Geometry: final body of the model. Coordinates: model frame, mm. Give positions to 0.01 mm unless a question says otherwise; leave off trailing zeros. Order: outer loops, then holes, each group sorted by start corner. A loop starts at its lowest first (then second) coordinate and runs counter-clockwise, first axis right, second up. Notation, with made-up numbers: (-38.5, -27.75) -> (-1.5, -27.75) arc R19 ccw to (-1.5, 1.25) -> close; hole circle Ø4 at (79.5, 29). An arc over 180 degrees is marked (long way). Write item = value, one per line.
```python
from build123d import *

# Parameters (mm, degrees)
SKETCH1_W           = 368.3
SKETCH1_H           = 127
SKETCH1_R           = 2.032
BOSS_EXTRUDE1_DEPTH = 3.175
FILLET1_R           = 5.08
FILLET3_R           = 6.35
FILLET4_R           = 2.54
FILLET5_R           = 6.35
CUT_EXTRUDE1_REACH  = 196.817
SKETCH2_R           = 2.032


with BuildPart() as part:
    # Sketch1 → Boss-Extrude1 (new body)
    with BuildSketch(Plane(origin=(0, 0, 0), x_dir=(1, 0, 0), z_dir=(0, 1, 0))):
        Rectangle(SKETCH1_W, SKETCH1_H)
        with Locations(Location((-171.45, -57.15, 0), (0, 0, 270))):
            Circle(SKETCH1_R, mode=Mode.SUBTRACT)
        with Locations(Location((-146.05, -57.15, 0), (0, 0, 270))):
            Circle(SKETCH1_R, mode=Mode.SUBTRACT)
        with Locations(Location((-95.25, -45.0215, 0), (0, 0, 270))):
            Circle(SKETCH1_R, mode=Mode.SUBTRACT)
        with Locations(Location((-82.55, -45.0215, 0), (0, 0, 270))):
            Circle(SKETCH1_R, mode=Mode.SUBTRACT)
        with Locations(Location((-60.9677978, -44.45, 0), (0, 0, 270))):
            Circle(SKETCH1_R, mode=Mode.SUBTRACT)
        with Locations(Location((-48.2677978, -44.45, 0), (0, 0, 270))):
            Circle(SKETCH1_R, mode=Mode.SUBTRACT)
        with Locations(Location((-154.94, -18.415, 0), (0, 0, 270))):
            Circle(SKETCH1_R, mode=Mode.SUBTRACT)
        with Locations(Location((-142.24, -18.415, 0), (0, 0, 270))):
            Circle(SKETCH1_R, mode=Mode.SUBTRACT)
        with Locations(Location((2.1088604, -44.45, 0), (0, 0, 270))):
            Circle(SKETCH1_R, mode=Mode.SUBTRACT)
        with Locations(Location((14.8088604, -44.45, 0), (0, 0, 270))):
            Circle(SKETCH1_R, mode=Mode.SUBTRACT)
        with Locations(Location((158.3188604, -44.45, 0), (0, 0, 270))):
            Circle(SKETCH1_R, mode=Mode.SUBTRACT)
        with Locations(Location((171.0188604, -44.45, 0), (0, 0, 270))):
            Circle(SKETCH1_R, mode=Mode.SUBTRACT)
        Polygon((-134.618428208, -13.335), (-165.098428208, -13.335), (-165.098428208, 40.005), (-134.618428208, 40.005), (-134.618428208, 26.67), (-126.998428208, 26.67), (-126.998428208, 0), (-134.618428208, 0), align=None, mode=Mode.SUBTRACT)
        with Locations(Location((-60.9677978, 0, 0), (0, 0, 270))):
            Circle(SKETCH1_R, mode=Mode.SUBTRACT)
        with Locations(Location((-48.2677978, 0, 0), (0, 0, 270))):
            Circle(SKETCH1_R, mode=Mode.SUBTRACT)
        with Locations(Location((-171.45, 57.15, 0), (0, 0, 270))):
            Circle(SKETCH1_R, mode=Mode.SUBTRACT)
        with Locations(Location((-146.05, 57.15, 0), (0, 0, 270))):
            Circle(SKETCH1_R, mode=Mode.SUBTRACT)
        with Locations(Location((-60.9677978, 44.45, 0), (0, 0, 270))):
            Circle(SKETCH1_R, mode=Mode.SUBTRACT)
        with Locations(Location((-48.2677978, 44.45, 0), (0, 0, 270))):
            Circle(SKETCH1_R, mode=Mode.SUBTRACT)
        with Locations(Location((2.1088604, 0, 0), (0, 0, 270))):
            Circle(SKETCH1_R, mode=Mode.SUBTRACT)
        with Locations(Location((14.8088604, 0, 0), (0, 0, 270))):
            Circle(SKETCH1_R, mode=Mode.SUBTRACT)
        with Locations(Location((158.3188604, 0, 0), (0, 0, 270))):
            Circle(SKETCH1_R, mode=Mode.SUBTRACT)
        with Locations(Location((171.0188604, 0, 0), (0, 0, 270))):
            Circle(SKETCH1_R, mode=Mode.SUBTRACT)
        with Locations(Location((2.1088604, 44.45, 0), (0, 0, 270))):
            Circle(SKETCH1_R, mode=Mode.SUBTRACT)
        with Locations(Location((14.8088604, 44.45, 0), (0, 0, 270))):
            Circle(SKETCH1_R, mode=Mode.SUBTRACT)
        with Locations(Location((158.3188604, 44.45, 0), (0, 0, 270))):
            Circle(SKETCH1_R, mode=Mode.SUBTRACT)
        with Locations(Location((171.0188604, 44.45, 0), (0, 0, 270))):
            Circle(SKETCH1_R, mode=Mode.SUBTRACT)
    extrude(amount=BOSS_EXTRUDE1_DEPTH)

    # Fillet1
    fillet1_edges = [part.edges().sort_by_distance(p)[0] for p in [
        (-134.618428208, 1.5875, -40.005),
        (-165.098428208, 1.5875, -40.005),
        (-165.098428208, 1.5875, 13.335),
        (-134.618428208, 1.5875, 13.335),
    ]]
    fillet(fillet1_edges, radius=FILLET1_R)

    # Fillet3
    fillet3_edges = [part.edges().sort_by_distance(p)[0] for p in [
        (184.15, 1.5875, -63.5),
        (184.15, 1.5875, 63.5),
        (-184.15, 1.5875, 63.5),
        (-184.15, 1.5875, -63.5),
    ]]
    fillet(fillet3_edges, radius=FILLET3_R)

    # Fillet4
    fillet4_edges = [part.edges().sort_by_distance(p)[0] for p in [
        (-126.998428208, 1.5875, -26.67),
        (-126.998428208, 1.5875, 0),
    ]]
    fillet(fillet4_edges, radius=FILLET4_R)

    # Fillet5
    fillet5_edges = [part.edges().sort_by_distance(p)[0] for p in [
        (-134.618428208, 1.5875, 0),
        (-134.618428208, 1.5875, -26.67),
    ]]
    fillet(fillet5_edges, radius=FILLET5_R)

    # Sketch2 → Cut-Extrude1 (cut, up to next)
    with BuildSketch(Plane(origin=(0, 3.175, 0), x_dir=(1, 0, 0), z_dir=(0, 1, 0)), mode=Mode.PRIVATE) as cut_extrude1_sk1:
        with Locations(Location((139.7, 22.86, 0), (0, 0, 270))):
            Circle(SKETCH2_R)
    cut_extrude1_tool1 = extrude(cut_extrude1_sk1.sketch, amount=-CUT_EXTRUDE1_REACH, mode=Mode.PRIVATE) & part.part
    # Sketch2 → Cut-Extrude1 (cut, up to next)
    with BuildSketch(Plane(origin=(0, 3.175, 0), x_dir=(1, 0, 0), z_dir=(0, 1, 0)), mode=Mode.PRIVATE) as cut_extrude1_sk2:
        with Locations(Location((139.7, 54.61, 0), (0, 0, 270))):
            Circle(SKETCH2_R)
    cut_extrude1_tool2 = extrude(cut_extrude1_sk2.sketch, amount=-CUT_EXTRUDE1_REACH, mode=Mode.PRIVATE) & part.part
    # Sketch2 → Cut-Extrude1 (cut, up to next)
    with BuildSketch(Plane(origin=(0, 3.175, 0), x_dir=(1, 0, 0), z_dir=(0, 1, 0)), mode=Mode.PRIVATE) as cut_extrude1_sk3:
        with Locations(Location((-22.86, 54.61, 0), (0, 0, 270))):
            Circle(SKETCH2_R)
    cut_extrude1_tool3 = extrude(cut_extrude1_sk3.sketch, amount=-CUT_EXTRUDE1_REACH, mode=Mode.PRIVATE) & part.part
    # Sketch2 → Cut-Extrude1 (cut, up to next)
    with BuildSketch(Plane(origin=(0, 3.175, 0), x_dir=(1, 0, 0), z_dir=(0, 1, 0)), mode=Mode.PRIVATE) as cut_extrude1_sk4:
        with Locations(Location((-22.86, 22.86, 0), (0, 0, 270))):
            Circle(SKETCH2_R)
    cut_extrude1_tool4 = extrude(cut_extrude1_sk4.sketch, amount=-CUT_EXTRUDE1_REACH, mode=Mode.PRIVATE) & part.part
    # Sketch2 → Cut-Extrude1 (cut, up to next)
    with BuildSketch(Plane(origin=(0, 3.175, 0), x_dir=(1, 0, 0), z_dir=(0, 1, 0)), mode=Mode.PRIVATE) as cut_extrude1_sk5:
        with Locations(Location((-107.95, 54.61, 0), (0, 0, 270))):
            Circle(SKETCH2_R)
    cut_extrude1_tool5 = extrude(cut_extrude1_sk5.sketch, amount=-CUT_EXTRUDE1_REACH, mode=Mode.PRIVATE) & part.part
    # Sketch2 → Cut-Extrude1 (cut, up to next)
    with BuildSketch(Plane(origin=(0, 3.175, 0), x_dir=(1, 0, 0), z_dir=(0, 1, 0)), mode=Mode.PRIVATE) as cut_extrude1_sk6:
        with Locations(Location((-107.95, 45.72, 0), (0, 0, 270))):
            Circle(SKETCH2_R)
    cut_extrude1_tool6 = extrude(cut_extrude1_sk6.sketch, amount=-CUT_EXTRUDE1_REACH, mode=Mode.PRIVATE) & part.part
    add(cut_extrude1_tool1.solids().sort_by_distance((139.7, 3.175, -22.86))[0], mode=Mode.SUBTRACT)
    add(cut_extrude1_tool2.solids().sort_by_distance((139.7, 3.175, -54.61))[0], mode=Mode.SUBTRACT)
    add(cut_extrude1_tool3.solids().sort_by_distance((-22.86, 3.175, -54.61))[0], mode=Mode.SUBTRACT)
    add(cut_extrude1_tool4.solids().sort_by_distance((-22.86, 3.175, -22.86))[0], mode=Mode.SUBTRACT)
    add(cut_extrude1_tool5.solids().sort_by_distance((-107.95, 3.175, -54.61))[0], mode=Mode.SUBTRACT)
    add(cut_extrude1_tool6.solids().sort_by_distance((-107.95, 3.175, -45.72))[0], mode=Mode.SUBTRACT)


solid = part.part
```
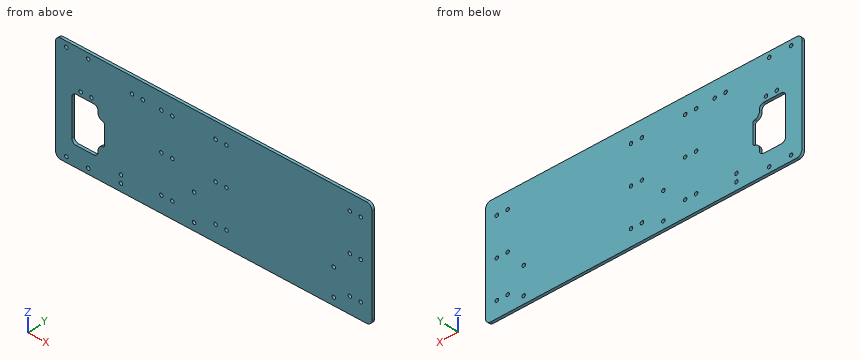
1) First-contact query: P1, Ø6, axis at x = 105, z = 15.5, coming from the -Y side; P2, Ø3.5, axis at x = 2.11, z = 0, coming from the +Y side. Flat tips, straight axial feed; report the tip coordinate or a pass-through.
Check sheet entries:
P1 = 0
P2 = through
2) Section query B-B (y = 1.15). Count the separate pieces of the cut face and the enclosed holes in it, plus the area to 3 significant figures.
Check sheet entries:
separate_pieces = 1
enclosed_holes = 33
area = 44,500 mm²
3) Line query: line 1 (Z direction, x = -146.05, y = 1.65) (3 decimals); line 2 (X direction, y = 0.7, z = -22.86); line 3 (Z direction, x = -159, y = 2.5) (3 decimals). Output: solid intervals per line, ascending. Write a range as from..to.
Check sheet entries:
line_1 = -63.5..-59.182, -55.118..-40.005, 13.335..55.118, 59.182..63.5
line_2 = -184.15..-165.1, -127..-24.89, -20.83..137.67, 141.73..184.15
line_3 = -63.5..-40.005, 13.335..63.5
4) Section query A-A (z = -13.5). Output: boundary loops of the cut face in (x, y) (3 decimals), plus the area to 3 significant figures.
Check sheet entries:
outline = (-184.15, 0) -> (-165.098, 0) -> (-165.098, 3.175) -> (-184.15, 3.175) -> close; (-126.998, 0) -> (184.15, 0) -> (184.15, 3.175) -> (-126.998, 3.175) -> close
area = 1,050 mm²
